Here's how the part is built. I have some questions about the finished solid (model axes, mm). Round coordinates to 2 decimals unless told otherwise and drop trailing zeros. Order: outer loops, then holes, each group sorted by start corner. A loop starts at its lowest first (then second) coordinate and runs counter-clockwise, first axis right, second up. Notation, with made-up numbers: (-17.75, 13.5) -> (35.25, 13.5) arc R8 cw to (35.25, 26.5) -> close; hole circle Ø3 at (-19, -28). An arc over 180 degrees is marked (long way). Answer in a Markdown table with one row per item.
```python
from build123d import *

# Parameters (mm, degrees)
SKETCH1_W           = 50
SKETCH1_H           = 15
BOSS_EXTRUDE1_DEPTH = 35
SKETCH2_R           = 2.5
CUT_EXTRUDE1_DEPTH  = 30
SKETCH3_R           = 5.055
BOSS_EXTRUDE2_DEPTH = 15


with BuildPart() as part:
    # Sketch1 → Boss-Extrude1 (new body)
    with BuildSketch(Plane.XY):
        Rectangle(SKETCH1_W, SKETCH1_H)
    extrude(amount=BOSS_EXTRUDE1_DEPTH)

    # Sketch2 → Cut-Extrude1 (cut)
    with BuildSketch(Plane(origin=(0, 7.5, 0), x_dir=(1, 0, 0), z_dir=(0, 1, 0))):
        with Locations(Location((17.5, -6.5, 0), (0, 0, 270))):
            Circle(SKETCH2_R)
        with Locations(Location((17.5, -28.5, 0), (0, 0, 270))):
            Circle(SKETCH2_R)
        with Locations(Location((-17.5, -28.5, 0), (0, 0, 270))):
            Circle(SKETCH2_R)
        with Locations(Location((-17.5, -6.5, 0), (0, 0, 270))):
            Circle(SKETCH2_R)
    extrude(amount=-CUT_EXTRUDE1_DEPTH, mode=Mode.SUBTRACT)

    # Sketch3 → Boss-Extrude2 (add)
    with BuildSketch(Plane.XY.offset(35)):
        Circle(SKETCH3_R)
    extrude(amount=BOSS_EXTRUDE2_DEPTH)


solid = part.part
```
1. Please list where these lines run through material, in increasing order: line 1 along X through (y, z) = (-5, 28.5); line 2 along Z through (x, y) = (-18, 0.25); line 3 along Z through (x, y) = (19, -3.5).
Numbers:
| item | result |
|---|---|
| line 1 | x = -25 to -20, -15 to 15, 20 to 25 |
| line 2 | z = 0 to 4.05, 8.95 to 26.05, 30.95 to 35 |
| line 3 | z = 0 to 4.5, 8.5 to 26.5, 30.5 to 35 |
2. Suppose I cut it at B-B on y = 0. Write out the boundary of the cut face in (x, z) (3 decimals).
Numbers:
| item | result |
|---|---|
| outline | (-25, 0) -> (25, 0) -> (25, 35) -> (5.055, 35) -> (5.055, 50) -> (-5.055, 50) -> (-5.055, 35) -> (-25, 35) -> close; hole circle Ø5 at (-17.5, 6.5); hole circle Ø5 at (-17.5, 28.5); hole circle Ø5 at (17.5, 6.5); hole circle Ø5 at (17.5, 28.5) |
3. For pin 1 Ø1.5 at (x, y) = (15.5, 2.5) entering from +Z; pin 2 Ø6 at (x, y) = (0.5, -2.5) entering from -Z, each with a flat end and sliding along its axis, tell me the tip position at first contact or that it passes through.
Numbers:
| item | result |
|---|---|
| pin 1 | stops at z = 35 |
| pin 2 | stops at z = 0 |
4. We'd pull the mould along Z, two halves only. Please class faces 1 (the face through (19.61, 0.11, 7.84)), 2 (the face through (-4.01, -3.08, 42.4)), 3 (the face through (-19, 0.1, 26.5)), 4 (the face through (0, 0, 50)): released by +Z, released by -Z, zero draft, split by the parting line, or undercut.
Numbers:
| item | result |
|---|---|
| face 1 | undercut |
| face 2 | zero draft |
| face 3 | undercut |
| face 4 | released by +Z |
5. Suppose I cut it at C-C on z = 6.5. Write out the boundary of the cut face in (x, y).
Numbers:
| item | result |
|---|---|
| outline | (-25, -7.5) -> (-20, -7.5) -> (-20, 7.5) -> (-25, 7.5) -> close; (-15, -7.5) -> (15, -7.5) -> (15, 7.5) -> (-15, 7.5) -> close; (20, -7.5) -> (25, -7.5) -> (25, 7.5) -> (20, 7.5) -> close |
6. Suppose I cut it at A-A on x = 17.5. Write out the boundary of the cut face in (y, z).
Numbers:
| item | result |
|---|---|
| outline | (-7.5, 0) -> (7.5, 0) -> (7.5, 4) -> (-7.5, 4) -> close; (-7.5, 9) -> (7.5, 9) -> (7.5, 26) -> (-7.5, 26) -> close; (-7.5, 31) -> (7.5, 31) -> (7.5, 35) -> (-7.5, 35) -> close |
7. Suppose I cut it at D-D on x = 0. Write out the boundary of the cut face in (y, z) (3 decimals), then the cut area to 3 significant figures.
Numbers:
| item | result |
|---|---|
| outline | (-7.5, 0) -> (7.5, 0) -> (7.5, 35) -> (5.055, 35) -> (5.055, 50) -> (-5.055, 50) -> (-5.055, 35) -> (-7.5, 35) -> close |
| area | 677 mm2 |
